For this review, take the finished solid that the model builds, in its own axes (mm). Face numbers are marked on the shaded views. A direction names the side the tool comes from. Coordinates: 2 decimals unless noted, no trailing zeros. Loops run counter-clockwise (first coordinate to the right, second up) from the corner with the lowest first, then second, coordinate; pieces in that order, holes last. Notation, with made-up numbers: M 37.5,-31 L 96.5,-31 A25 cw 96.5,-19 Z; hole C 80.25,40.25 d5. An arc over 180 degrees is marked long. Put each result on its own line as item: value.
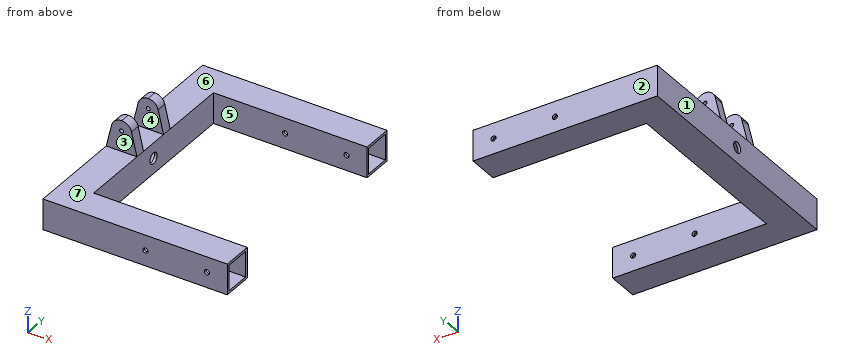
```python
from build123d import *

# Parameters (mm, degrees)
F1_DEPTH = 76.2
F2_T     = -6.35
F4_D     = 12.7
F7_DEPTH = 12.7
F8_R     = 13.4197326433
F9_DEPTH = 228.601


# Not quite as in the source:
# - a feature names something its author has since deleted; it is built from what else it names


with BuildPart() as f1:
    # F0 (on Top) → F1 (new body)
    with BuildSketch(Plane.XY):
        Polygon((-228.6, 304.8), (-228.6, -304.8), (228.6, -304.8), (228.6, -228.6), (-152.4, -228.6), (-152.4, 228.6), (228.6, 228.6), (228.6, 304.8), align=None)
    extrude(amount=F1_DEPTH)

    # F2
    f2_openings = [f1.faces().sort_by_distance(p)[0] for p in [
        (228.6, -266.7, 38.1),
        (228.6, 266.7, 38.1),
    ]]
    offset(amount=F2_T, openings=f2_openings, kind=Kind.INTERSECTION)

    # F4 (through all)
    with Locations(Plane(origin=(0, 304.8, 0), x_dir=(-1, 0, 0), z_dir=(0, 1, 0))):
        with Locations((-177.8, 38.1), (-25.4, 38.1)):
            Hole(F4_D / 2)

    # F6 (on offset) → F7 (join, symmetric)
    with BuildSketch(Plane.XZ.offset(50.8)):
        with BuildLine():
            Line((-215.2195876243, 132.8396907182), (-228.6, 76.2))
            Line((-228.6, 76.2), (-190.5, 76.2))
            Line((-190.5, 76.2), (-190.5, 122.2375))
            ThreePointArc((-190.5, 122.2375), (-195.2625, 127), (-190.5, 131.7625))
            Line((-190.5, 131.7625), (-190.5, 152.4))
            ThreePointArc((-190.5, 152.4), (-206.2612159391, 146.9184354838), (-215.2195876243, 132.8396907182))
        make_face()
        with BuildLine():
            Line((-190.5, 122.2375), (-190.5, 76.2))
            Line((-190.5, 76.2), (-152.4, 76.2))
            Line((-152.4, 76.2), (-165.7804123757, 132.8396907182))
            ThreePointArc((-165.7804123757, 132.8396907182), (-174.7387840609, 146.9184354838), (-190.5, 152.4))
            Line((-190.5, 152.4), (-190.5, 131.7625))
            ThreePointArc((-190.5, 131.7625), (-187.1324039546, 130.3675960454), (-185.7375, 127))
            ThreePointArc((-185.7375, 127), (-187.1324039546, 123.6324039546), (-190.5, 122.2375))
        make_face()
    extrude(amount=F7_DEPTH, both=True)

    # F8 (on Right) → F9 (cut, through all)
    with BuildSketch(Plane.YZ):
        with Locations((0, 38.1)):
            Circle(F8_R)
    extrude(amount=-F9_DEPTH, mode=Mode.SUBTRACT)

    # F10: F1 across plane


with BuildPart() as f1_1:
    add(f1.part)
    add(f1.part.mirror(Plane.XZ))


solid = f1_1.part
```
(1) Add section B-B (y = 0). Write out the cut boundary in (x, z).
Determined:
outline: M -228.6,0 L -152.4,0 L -152.4,24.68 L -158.75,24.68 L -158.75,6.35 L -222.25,6.35 L -222.25,24.68 L -228.6,24.68 Z; M -228.6,51.52 L -222.25,51.52 L -222.25,69.85 L -158.75,69.85 L -158.75,51.52 L -152.4,51.52 L -152.4,76.2 L -228.6,76.2 Z
(2) Add section A-A (x = -84). Write out the cut boundary in (y, z), plus the area to 3 significant figures.
Determined:
outline: M -304.8,0 L -228.6,0 L -228.6,76.2 L -304.8,76.2 Z; M 228.6,0 L 304.8,0 L 304.8,76.2 L 228.6,76.2 Z; hole M -298.45,6.35 L -234.95,6.35 L -234.95,69.85 L -298.45,69.85 Z; hole M 234.95,6.35 L 298.45,6.35 L 298.45,69.85 L 234.95,69.85 Z
area: 3,550 mm^2
(3) Wall thickness on line 1 along Y through (x, z) = (-71, 14.5); line 2 along Z through (x, y) = (-190, -58); line 3 along X through (y, z) = (-301, 38): over which ranges is each line inside the solid? List them lowest first. Write a range as [from, to].
Determined:
line 1: y = [-304.8, -298.45], [-234.95, -228.6], [228.6, 234.95], [298.45, 304.8]
line 2: z = [0, 6.35], [69.85, 122.26], [131.74, 152.4]
line 3: x = [-228.6, 19.05], [31.75, 171.45], [184.15, 228.6]
(4) Add section D-D (z = 111.5). Write out the cut boundary in (x, y).
Determined:
outline: M -220.26,-63.5 L -160.74,-63.5 L -160.74,-38.1 L -220.26,-38.1 Z; M -220.26,38.1 L -160.74,38.1 L -160.74,63.5 L -220.26,63.5 Z
(5) Draft analysis for pull direction Y (two halves, no side actions). For the marked faces 1, 2, 3 and 4, state which applies: +Y half, -Y half, draft (parallel to the pull), parting line (faces both ways), or undercut.
Determined:
face 1: draft
face 2: +Y half
face 3: -Y half
face 4: undercut
(6) Add section C-C (x = 25.4). State how many separate pieces and enclosed holes the cut face has, plus the area to 3 significant figures.
Determined:
separate pieces: 4
enclosed holes: 0
area: 3,230 mm^2
(7) Tool access review of the marked faces 5, 6 and 7: name each direction out of +Z, -Z, +X, -X, +Y, -Y from which nothing blocks a thin tool from reaching the whole face with its end or side.
Determined:
face 5: +Z, -Z, +X
face 6: +Z, +X, -X, +Y
face 7: +Z, +X, -X, -Y
(8) For pin 1 (5.5 mm diameter, centred on x = -190.5, z = 127, fed in from +Y); pin 2 (16.5 mm diameter, centred on x = 177.8, z = 38.1, fed in from -Y); pin 3 (12 mm diameter, centred on x = -179.5, y = -61.5, fed in from +Z), all flat-tipped, find the tip position at first contact; note any pin that passes through.
Determined:
pin 1: passes through
pin 2: stops at y = -304.8
pin 3: stops at z = 151.9
